```python
from build123d import *

# Parameters (mm, degrees)
SKETCH_1_W          = 30
SKETCH_1_H          = 15
EXTRUDE_1_DEPTH     = 4
SKETCH_2_W          = 45
SKETCH_2_H          = 2.5
EXTRUDE_2_DEPTH     = 13
SKETCH_3_R          = 1.5
CUT_EXTRUDE_1_DEPTH = 25
FILLET_1_R          = 3
SKETCH_4_R          = 1.5
CUT_EXTRUDE_2_DEPTH = 25
SKETCH_5_R          = 3.5
CUT_EXTRUDE_3_DEPTH = 2
FILLET_2_R          = 5
SKETCH_6_RX         = 8.962094073
SKETCH_6_RY         = 3.777931928
CUT_EXTRUDE_4_DEPTH = 10
SKETCH_7_R          = 4
CUT_EXTRUDE_5_DEPTH = 10


with BuildPart() as part:
    # 草图1 → 凸台-拉伸1 (new body)
    with BuildSketch(Plane(origin=(0, 0, 0), x_dir=(1, 0, 0), z_dir=(0, 1, 0))):
        Rectangle(SKETCH_1_W, SKETCH_1_H)
    extrude(amount=EXTRUDE_1_DEPTH)

    # 草图2 → 凸台-拉伸2 (add)
    with BuildSketch(Plane(origin=(0, 4, 0), x_dir=(1, 0, 0), z_dir=(0, 1, 0))):
        with Locations((0, 6.25)):
            Rectangle(SKETCH_2_W, SKETCH_2_H)
    extrude(amount=EXTRUDE_2_DEPTH)

    # 草图3 → 切除-拉伸1 (cut)
    with BuildSketch(Plane.XY.offset(-5)):
        with Locations((18.75, 10.5)):
            Circle(SKETCH_3_R)
        with Locations((-18.75, 10.5)):
            Circle(SKETCH_3_R)
    extrude(amount=-CUT_EXTRUDE_1_DEPTH, mode=Mode.SUBTRACT)

    # 圆角1
    fillet_1_edges = [part.edges().sort_by_distance(p)[0] for p in [
        (-15, 2, 7.5),
        (15, 2, 7.5),
        (15, 4, -6.25),
        (-15, 4, -6.25),
        (-22.5, 17, -6.25),
        (22.5, 17, -6.25),
    ]]
    fillet(fillet_1_edges, radius=FILLET_1_R)

    # 草图4 → 切除-拉伸2 (cut)
    with BuildSketch(Plane(origin=(0, 4, 0), x_dir=(1, 0, 0), z_dir=(0, 1, 0))):
        with Locations(Location((10, 0, 0), (0, 0, 270))):
            Circle(SKETCH_4_R)
        with Locations(Location((-10, 0, 0), (0, 0, 270))):
            Circle(SKETCH_4_R)
    extrude(amount=-CUT_EXTRUDE_2_DEPTH, mode=Mode.SUBTRACT)

    # 草图5 → 切除-拉伸3 (cut)
    with BuildSketch(Plane(origin=(0, 4, 0), x_dir=(1, 0, 0), z_dir=(0, 1, 0))):
        with Locations(Location((10, 0, 0), (0, 0, 270))):
            Circle(SKETCH_5_R)
        with Locations(Location((-10, 0, 0), (0, 0, 270))):
            Circle(SKETCH_5_R)
    extrude(amount=-CUT_EXTRUDE_3_DEPTH, mode=Mode.SUBTRACT)

    # 圆角2
    fillet_2_edges = [part.edges().sort_by_distance(p)[0] for p in [
        (-22.5, 4, -6.25),
        (22.5, 4, -6.25),
    ]]
    fillet(fillet_2_edges, radius=FILLET_2_R)

    # 草图6 → 切除-拉伸4 (cut)
    with BuildSketch(Plane.XY.offset(-5)):
        with Locations((0, 10.28402341)):
            Ellipse(SKETCH_6_RX, SKETCH_6_RY)
    extrude(amount=-CUT_EXTRUDE_4_DEPTH, mode=Mode.SUBTRACT)

    # 草图7 → 切除-拉伸5 (cut)
    with BuildSketch(Plane(origin=(0, 4, 0), x_dir=(1, 0, 0), z_dir=(0, 1, 0))):
        with Locations(Location((0, -1.406230218, 0), (0, 0, 270))):
            Circle(SKETCH_7_R)
    extrude(amount=-CUT_EXTRUDE_5_DEPTH, mode=Mode.SUBTRACT)


solid = part.part
```
Build history of the part. All positions in model axes, mm. A direction names the side the tool comes from. Coordinates: 2 decimals unless noted, no trailing zeros. Order: outer loops, then holes, each group sorted by start corner. A loop starts at its lowest first (then second) coordinate and runs counter-clockwise, first axis right, second up. Notation, with made-up numbers: (43.5, -31) -> (59.5, -31) arc R28 ccw to (59.5, -3) -> close; hole circle Ø4 at (88.25, 23). An arc over 180 degrees is marked (long way). Answer in a Markdown table with one row per item. Add a question column.
Q1. Mould opens along Z. For faces 1 (the face through (-0.31, 14.22, -5)), 2 (the face through (-11.464, 1.014, -0.325)), 3 (the face through (-22.5, 11, -6)) say: +Z half, -Z half, draft (parallel to the pull), parting line (faces both ways), or undercut.
Q2. Band-saw the part on B-B, the plane z = 0. List the corners of the cut face in (x, y), then the cut area to 3 significant figures.
Q3. Band-saw the part on A-A, the plane x = 10. List the corners of the cut face in (y, z), then the cut area to 3 significant figures.
Q4. Which spindle directions (+Z, -Z, +X, -X, +Y, -Y) get a long thin tool onto all of the face, cutting with end or side? Do faces 4 (the face through (10, 2, 2)), 5 (the face through (-2.43, 2.03, -1.77)). Say none if no direction does.
Q5. Drop flat-ended pins along their axis: pin 1 (2.5 mm diameter, centred on x = 18.75, y = 10.5, fed in from +Z); pin 2 (5.5 mm diameter, centred on x = -9, z = 0, fed in from +Y); pin 3 (4 mm diameter, centred on x = 10, z = 0, fed in from +Y); pin 4 (1.2 mm diameter, centred on y = 1.5, z = 0, fed in from +X). Give the stop position or say it passes through.
Q6. Wall check: line 1 along Z through (x, y) = (-6, 14.25); line 2 along Y through (x, z) = (5.5, -1.75); line 3 along X through (y, z) = (1.25, 0). Give the ranges that are in metal, low to high. Write a range as [from, to].
Q7. Band-saw the part on C-C, the plane x = 0. Give the number of separate pieces and of enclosed holes in the cut face, then the cut area to 3 significant figures.
Answers follow:
| question | item | result |
|---|---|---|
| 1 | face 1 | +Z half |
| 1 | face 2 | undercut |
| 1 | face 3 | draft |
| 2 | outline | (-15, 0) -> (-11.5, 0) -> (-11.5, 2) -> (-13.5, 2) -> (-13.5, 4) -> (-15, 4) -> close; (-8.5, 0) -> (-3.74, 0) -> (-3.74, 4) -> (-6.5, 4) -> (-6.5, 2) -> (-8.5, 2) -> close; (3.74, 0) -> (8.5, 0) -> (8.5, 2) -> (6.5, 2) -> (6.5, 4) -> (3.74, 4) -> close; (11.5, 0) -> (15, 0) -> (15, 4) -> (13.5, 4) -> (13.5, 2) -> (11.5, 2) -> close |
| 2 | area | 50.0 mm^2 |
| 3 | outline | (0, -7.5) -> (17, -7.5) -> (17, -5) -> (4, -5) -> (4, -3.5) -> (2, -3.5) -> (2, -1.5) -> (0, -1.5) -> close; (0, 1.5) -> (2, 1.5) -> (2, 3.5) -> (4, 3.5) -> (4, 7.5) -> (0, 7.5) -> close |
| 3 | area | 72.5 mm^2 |
| 4 | face 4 | +Y |
| 4 | face 5 | +Y, -Y |
| 5 | pin 1 | through |
| 5 | pin 2 | y = 4 |
| 5 | pin 3 | y = 2 |
| 5 | pin 4 | x = 15 |
| 6 | line 1 | [-7.5, -5] |
| 6 | line 2 | [0, 4] |
| 6 | line 3 | [-15, -11.5], [-8.5, -3.74], [3.74, 8.5], [11.5, 15] |
| 7 | separate pieces | 3 |
| 7 | enclosed holes | 0 |
| 7 | area | 41.6 mm^2 |
